Can you work these out from the model? Positions are in its coordinate system, mm. Face numbers are marked on the shaded views. A direction names the side the tool comes from. Coordinates: 2 decimals unless noted, no trailing zeros. Order: outer loops, then holes, each group sorted by start corner. A loop starts at its lowest first (then second) coordinate and runs counter-clockwise, first axis right, second up. Notation, with made-up numbers: (18, -22) -> (73, -22) arc R22 cw to (73, -5) -> close; hole circle Ø6 at (18, 81.5). An arc over 180 degrees is marked (long way). Answer as a JSON object with one key per item and string values. Group by question number.
(1) I want a section at B-B, the plane x = 4.25. List the corners of the cut face in (y, z) for me.
(2) I need wall thicknesses on line 1 (Y direction, x = 4.75, z = 2.6); line 2 (X direction, y = 3.5, z = 1); line 3 (Y direction, x = 4, z = 1.1). Which ranges of each line are inside material? Lowest first, please.
(3) I want a section at C-C, the plane z = 2.05. List the corners of the cut face in (x, y) for me.
(4) I want a section at A-A, the plane y = 0. List the corners of the cut face in (x, z) for me, plus the area to 3 significant figures.
(5) For pin 1 (4 mm diameter, centred on x = -1.5, y = -3.5, fed in from +Z); pin 2 (2.5 mm diameter, centred on x = 4.56, y = -3.07, fed in from -Z); pin 3 (1.5 mm diameter, centred on y = 2.5, z = 3.5, fed in from +X); pin 4 (2 mm diameter, centred on x = -1.5, z = 2.5, fed in from +Y), each with a flat end and sliding along its axis, tell me the tip position at first contact or that it passes through.
(6) Which directions (+Z, -Z, +X, -X, +Y, -Y) give clear straight access to the entire face, cutting with the end or side of a thin tool? Please do the marked faces 1 and 2.
(7) If we mould it in two halves opening along Y, with no side actions, what happens to the marked faces 3, 4, 5 and 6? For each: pulls with the +Y half, pulls with the -Y half, needs draft (parallel to the pull), parting line crosses it, or undercut.
(8) I want a section at D-D, the plane x = 1.5. List the corners of the cut face in (y, z) for me.
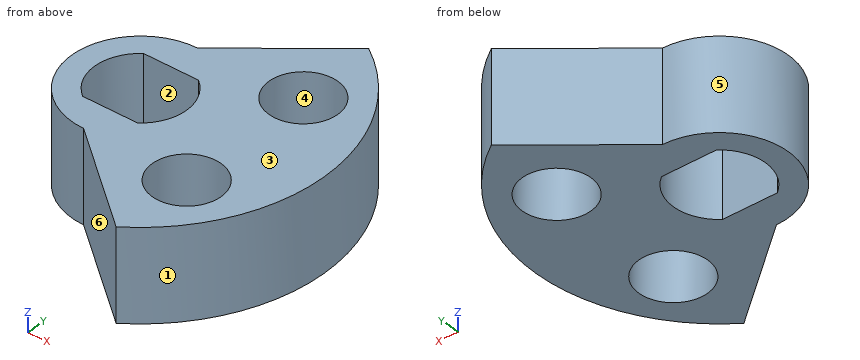
from build123d import *

# Parameters (mm, degrees)
F0_R     = 1.5
F1_DEPTH = 4


with BuildPart() as f1:
    # F0 (on Top) → F1 (new body)
    with BuildSketch(Plane.XY):
        with BuildLine():
            ThreePointArc((0, 3), (2.12132, 2.12132), (3, 0))
            ThreePointArc((3, 0), (2.12132, -2.12132), (0, -3))
            Line((0, -3), (4.448474, -6.649141))
            ThreePointArc((4.448474, -6.649141), (8, 0), (4.448474, 6.649141))
            Line((4.448474, 6.649141), (0, 3))
        make_face()
        with Locations((4.562768, -3.071017)):
            Circle(F0_R, mode=Mode.SUBTRACT)
        with Locations((4.562768, 3.071017)):
            Circle(F0_R, mode=Mode.SUBTRACT)
        with BuildLine():
            ThreePointArc((0, -3), (2.12132, -2.12132), (3, 0))
            ThreePointArc((3, 0), (2.12132, 2.12132), (0, 3))
            ThreePointArc((0, 3), (-3, 0), (0, -3))
        make_face()
        with BuildLine():
            ThreePointArc((1.2, 1.6), (2, 0), (1.2, -1.6))
            Line((1.2, -1.6), (-1.2, -1.6))
            ThreePointArc((-1.2, -1.6), (-2, 0), (-1.2, 1.6))
            Line((-1.2, 1.6), (1.2, 1.6))
        make_face(mode=Mode.SUBTRACT)
    extrude(amount=F1_DEPTH)


solid = f1.part
Computed values:
{
 "1": {"outline": "(-6.49, 0) -> (-4.54, 0) -> (-4.54, 4) -> (-6.49, 4) -> close; (-1.6, 0) -> (1.6, 0) -> (1.6, 4) -> (-1.6, 4) -> close; (4.54, 0) -> (6.49, 0) -> (6.49, 4) -> (4.54, 4) -> close"},
 "2": {"line 1": "y = -6.44 to -4.56, -1.58 to 1.58, 4.56 to 6.44", "line 2": "x = 0.61 to 3.13, 6 to 7.19", "line 3": "y = -6.28 to -4.46, -1.68 to 1.68, 4.46 to 6.28"},
 "3": {"outline": "(0, -3) -> (4.45, -6.65) arc R8 ccw to (4.45, 6.65) -> (0, 3) arc R3 ccw to start; hole (-1.2, -1.6) -> (1.2, -1.6) arc R2 ccw to (1.2, 1.6) -> (-1.2, 1.6) arc R2 ccw to start; hole circle Ø3 at (4.56, -3.07); hole circle Ø3 at (4.56, 3.07)"},
 "4": {"outline": "(-3, 0) -> (-2, 0) -> (-2, 4) -> (-3, 4) -> close; (2, 0) -> (8, 0) -> (8, 4) -> (2, 4) -> close", "area": "28.0 mm2"},
 "5": {"pin 1": "stops at z = 4", "pin 2": "passes through", "pin 3": "stops at x = 7.81", "pin 4": "stops at y = 2.96"},
 "6": {"face 1": "+Z, -Z, +X", "face 2": "+Z, -Z"},
 "7": {"face 3": "needs draft", "face 4": "undercut", "face 5": "parting line crosses it", "face 6": "pulls with the -Y half"},
 "8": {"outline": "(-4.23, 0) -> (-1.32, 0) -> (-1.32, 4) -> (-4.23, 4) -> close; (1.32, 0) -> (4.23, 0) -> (4.23, 4) -> (1.32, 4) -> close"}
}
